The model under review builds one solid part; all positions refer to its coordinate system, in mm. Give positions to 0.01 mm unless a question says otherwise; leave off trailing zeros. Order: outer loops, then holes, each group sorted by start corner. A loop starts at its lowest first (then second) coordinate and runs counter-clockwise, first axis right, second up.
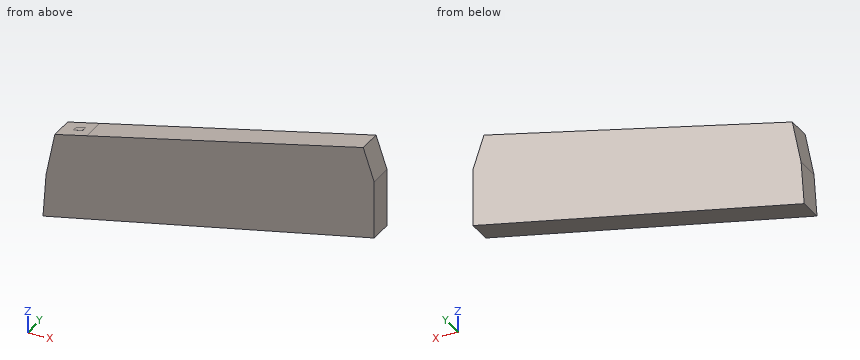
```python
from build123d import *

# Parameters (mm, degrees)
F1_DEPTH = 25.4
F2_W     = 10.3561803699
F2_H     = 5.641033873
F3_DEPTH = 0.0254


with BuildPart() as f1:
    # F0 (on Front) → F1 (new body)
    with BuildSketch(Plane.XZ):
        Polygon((-180.321587468, 14.7963562756), (-183.6662888527, -33.3735458553), (179.340466857, 53.3933117986), (179.340466857, 117.1431019902), (131.396189332, 143.0117189884), (-135.7338540163, 72.5921073616), (-170.688867569, 63.3774250746), align=None)
        Polygon((131.396189332, 143.0117189884), (179.340466857, 117.1431019902), (167.3504786853, 152.4898258342), align=None)
    extrude(amount=F1_DEPTH)

    # F2 (on face) → F3 (join)
    with BuildSketch(Plane(origin=(-26.7126271231, 0, 101.331789206), x_dir=(0.9669655535, 0, 0.2549070778), z_dir=(-0.2549070778, 0, 0.9669655535))):
        with Locations((-128.4218169749, -12.583672069)):
            Rectangle(F2_W, F2_H)
    extrude(amount=F3_DEPTH)


solid = f1.part
```
1. To check wall thickness, follow line 1 (Z direction, x = 62.5, y = -21.5); line 2 (Z direction, x = -103.5, y = -19.5); line 3 (X direction, y = -18, z = 59.5). State the ranges of each line that lie inside material, in increasing order.
2. Take a section at B-B (x = 155.5). Write out the cut boundary in (y, z).
3. Take a section at C-C (z = 84). Write out the cut boundary in (x, y).
4. Insertion check: pin 1 (12 mm diameter, centred on x = 46.5, y = -15, fed in from -Z); pin 2 (3 mm diameter, centred on x = -148.5, z = 68.5, fed in from +Y); pin 3 (2 mm diameter, centred on x = 54.5, y = -21, fed in from -Z); pin 4 (4 mm diameter, centred on x = -100.5, y = -4, fed in from -Z). Each pin has a flat end and moves straight along its axis. Give the tip position at first contact, or say it passes through.
5. Take a section at A-A (y = -5.75). Write out the cut boundary in (x, z), and give its area (3 significant figures).
Answer:
1. line 1: z = 25.47 to 124.85
1. line 2: z = -14.21 to 81.09
1. line 3: x = -171.46 to 179.34
2. outline: (-25.4, 47.69) - (0, 47.69) - (0, 149.37) - (-25.4, 149.37) - close
3. outline: (-92.46, -25.4) - (179.34, -25.4) - (179.34, 0) - (-92.46, 0) - close
4. pin 1: stops at z = 20.21
4. pin 2: stops at y = 0
4. pin 3: stops at z = 23.31
4. pin 4: stops at z = -13.97
5. outline: (-183.67, -33.37) - (179.34, 53.39) - (179.34, 117.14) - (167.35, 152.49) - (-170.69, 63.38) - (-180.32, 14.8) - close
5. area: 34,800 mm2
